Part print with two shaded views. Sizes in mm from the minimum x, y, z corner. Coordinates: 2 decimals unless noted, no trailing zeros. Order: outer loops, then holes, each group sorted by start corner. A loop starts at its lowest first (then second) coordinate and runs counter-clockwise, first axis right, second up. Notation, with made-up numbers: (0.25, 19.5) - (33.25, 19.5) arc R24 cw to (33.25, 50.5) - close; hole circle Ø8 at (-28.5, -30.75). An arc over 180 degrees is marked (long way). Return JSON: item names as keys, results as strings.
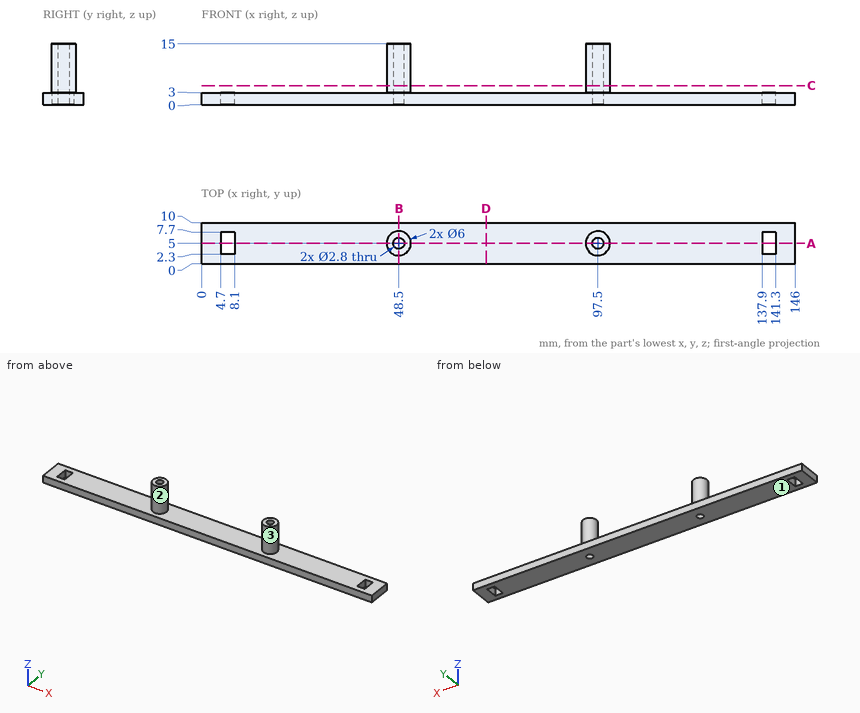
Item 1: Wall check: L1, parallel to Y at x = 97.5, z = 5.5; L2, parallel to X at y = 5.25, z = 12.75; L3, parallel to X at y = 5.5, z = 9.5. Give the ranges that are in metal, low to high. Write a range as [from, to].
Findings below:
{"L1": "y = [2, 3.6], [6.4, 8]", "L2": "x = [45.51, 47.12], [49.88, 51.49], [94.51, 96.12], [98.88, 100.49]", "L3": "x = [45.54, 47.19], [49.81, 51.46], [94.54, 96.19], [98.81, 100.46]"}
Item 2: Band-saw the part on A-A, the plane y = 5. List the corners of the cut face in (x, z), then the cut area to 3 significant figures.
Findings below:
{"outline": "(0, 0) - (4.7, 0) - (4.7, 3) - (0, 3) - close; (8.1, 0) - (47.1, 0) - (47.1, 15) - (45.5, 15) - (45.5, 3) - (8.1, 3) - close; (49.9, 0) - (96.1, 0) - (96.1, 15) - (94.5, 15) - (94.5, 3) - (51.5, 3) - (51.5, 15) - (49.9, 15) - close; (98.9, 0) - (137.9, 0) - (137.9, 3) - (100.5, 3) - (100.5, 15) - (98.9, 15) - close; (141.3, 0) - (146, 0) - (146, 3) - (141.3, 3) - close", "area": "478 mm²"}
Item 3: Band-saw the part on C-C, the plane z = 4.75. List the corners of the cut face in (x, y).
Findings below:
{"outline": "circle Ø6 at (48.5, 5); circle Ø6 at (97.5, 5); hole circle Ø2.8 at (48.5, 5); hole circle Ø2.8 at (97.5, 5)"}
Item 4: Mould opens along X. For the marked faces 1, 2 and 3 say: released by +X, released by -X, zero draft, split by the parting line, or undercut.
Findings below:
{"face 1": "zero draft", "face 2": "undercut", "face 3": "undercut"}
Item 5: Band-saw the part on D-D, the plane x = 70. List the corners of the cut face in (y, z).
Findings below:
{"outline": "(0, 0) - (10, 0) - (10, 3) - (0, 3) - close"}
Item 6: Drop flat-ended pins along their axis: P1, Ø4, axis at y = 8.5, z = 10.5, coming from the +X side; P2, Ø3, axis at y = 8, z = 11, coming from the -X side. Give the stop position or say it passes through.
Findings below:
{"P1": "stops at x = 100.1", "P2": "stops at x = 45.9"}
Item 7: Band-saw the part on B-B, the plane x = 48.5. List the corners of the cut face in (y, z), then the cut area to 3 significant figures.
Findings below:
{"outline": "(0, 0) - (3.6, 0) - (3.6, 15) - (2, 15) - (2, 3) - (0, 3) - close; (6.4, 0) - (10, 0) - (10, 3) - (8, 3) - (8, 15) - (6.4, 15) - close", "area": "60.0 mm²"}
